Check sheet for the modelled part. Datum: model origin and axes. Units: mm. A direction names the side the tool comes from. Give positions to 0.01 mm unless a question says otherwise; leave off trailing zeros. Write each loop counter-clockwise with the first axis right and the second up, starting at its lowest first coordinate (ties: lowest second). Pieces come first, ordered by that corner, then holes.
from build123d import *

# Parameters (mm, degrees)
SKETCH1_W               = 28
SKETCH1_H               = 17.5
PCB_DEPTH               = 1.6
MOUNT_HOLE_1_DEPTH      = 34.057676869
MOUNT_HOLE_1_DEPTH_BACK = 34.057676869
SKETCH2_R               = 1.5
MOUNT_HOLE_2_DEPTH      = 34.057676869
MOUNT_HOLE_2_DEPTH_BACK = 34.057676869
SKETCH3_R               = 1.5
HEADER_10PIN_START      = 1.6
SKETCH4_W               = 25.4
SKETCH4_H               = 2.5
HEADER_10PIN_DEPTH      = 8.5
ADS1115_IC_START        = 1.6
SKETCH5_W               = 5
SKETCH5_H               = 3
ADS1115_IC_DEPTH        = 1
CAPS_START              = 1.6
SKETCH6_W               = 2
SKETCH6_H               = 1.2
CAPS_DEPTH              = 0.8


with BuildPart() as part:
    # Sketch1 → PCB (new body)
    with BuildSketch(Plane(origin=(0, 0, 0), x_dir=(1, 0, 0), z_dir=(0, 1, 0))):
        with Locations((14, 8.75)):
            Rectangle(SKETCH1_W, SKETCH1_H)
    extrude(amount=PCB_DEPTH)

    # Sketch2 → Mount_hole_1 (cut, two sides: drawn at the far end of the back side and taken through both)
    with BuildSketch(Plane(origin=(0, 0, 0), x_dir=(1, 0, 0), z_dir=(0, 1, 0)).offset(-MOUNT_HOLE_1_DEPTH_BACK)):
        with Locations(Location((2.5, 15, 0), (0, 0, 270))):
            Circle(SKETCH2_R)
    extrude(amount=MOUNT_HOLE_1_DEPTH + MOUNT_HOLE_1_DEPTH_BACK, mode=Mode.SUBTRACT)

    # Sketch3 → Mount_hole_2 (cut, two sides: drawn at the far end of the back side and taken through both)
    with BuildSketch(Plane(origin=(0, 0, 0), x_dir=(1, 0, 0), z_dir=(0, 1, 0)).offset(-MOUNT_HOLE_2_DEPTH_BACK)):
        with Locations(Location((25.5, 15, 0), (0, 0, 270))):
            Circle(SKETCH3_R)
    extrude(amount=MOUNT_HOLE_2_DEPTH + MOUNT_HOLE_2_DEPTH_BACK, mode=Mode.SUBTRACT)

    # Sketch4 → Header_10pin (add)
    with BuildSketch(Plane(origin=(0, 0, 0), x_dir=(1, 0, 0), z_dir=(0, 1, 0)).offset(HEADER_10PIN_START)):
        with Locations((14, 1.65)):
            Rectangle(SKETCH4_W, SKETCH4_H)
    extrude(amount=HEADER_10PIN_DEPTH)

    # Sketch5 → ADS1115_IC (add)
    with BuildSketch(Plane(origin=(0, 0, 0), x_dir=(1, 0, 0), z_dir=(0, 1, 0)).offset(ADS1115_IC_START)):
        with Locations((13.5, 8)):
            Rectangle(SKETCH5_W, SKETCH5_H)
    extrude(amount=ADS1115_IC_DEPTH)

    # Sketch6 → Caps (add)
    with BuildSketch(Plane(origin=(0, 0, 0), x_dir=(1, 0, 0), z_dir=(0, 1, 0)).offset(CAPS_START)):
        with Locations((18.5, 7.1)):
            Rectangle(SKETCH6_W, SKETCH6_H)
    extrude(amount=CAPS_DEPTH)


solid = part.part
1) Draft check along X on faces 1 (the flat face through (18, 2, -7.7)), 2 (the flat face through (17.5, 2, -7)), 3 (the flat face through (11, 2, -8)). Enter one of: +X half, -X half, draft (parallel to the pull), parting line (faces both ways), or undercut.
2) Sectioned sample at C-C on y = 1.25. Record the boundary of the cut face in (x, z), then the cut area to 3 significant figures.
3) Scan lines: L1, parallel to X at y = 0.5, z = -15; L2, parallel to Z at x = 2.5, y = 0.95; L3, parallel to Y at x = 11.75, z = -7.5. Record each from-to range of solid material in increasing order.
4) Gauge pin test, flat ends, axial feed: pin 1 (1.2 mm diameter, centred on y = 6, z = -1.5, fed in from -X); pin 2 (2.5 mm diameter, centred on x = 13.5, z = -7.5, fed in from +Y); pin 3 (0.6 mm diameter, centred on x = 18.5, z = -7, fed in from +Y); pin 4 (2.5 mm diameter, centred on x = 2.5, z = -15, fed in from +Y). Record the tip position at first contact, or that the pin passes through.
5) Access from +Z, -Z, +X, -X, +Y, -Y to the whole of each face (thin tool, end or side, straight path). Record for faces 4 (the flat face through (13, 2.6, -8)), 5 (the flat face through (19.5, 2, -7)), 6 (the flat face through (1.3, 6, -2)), 7 (the flat face through (14, 6, -0.4)), 8 (the flat face through (26.7, 6, -2)).
6) Sectioned sample at A-A on x = 2.5. Record the boundary of the cut face in (y, z).
7) Sectioned sample at D-D on x = 19. Record the boundary of the cut face in (y, z), then the cut area to 3 significant figures.
8) Sectioned sample at B-B on z = -15. Record the boundary of the cut face in (x, y), then the cut area to 3 significant figures.
Answers below:
1. face 1: draft
1. face 2: undercut
1. face 3: -X half
2. outline: (0, -17.5) - (28, -17.5) - (28, 0) - (0, 0) - close; hole circle Ø3 at (2.5, -15); hole circle Ø3 at (25.5, -15)
2. area: 476 mm2
3. L1: x = 0 to 1, 4 to 24, 27 to 28
3. L2: z = -17.5 to -16.5, -13.5 to 0
3. L3: y = 0 to 2.6
4. pin 1: stops at x = 1.3
4. pin 2: stops at y = 2.6
4. pin 3: stops at y = 2.4
4. pin 4: passes through
5. face 4: -Z, +X, -X, +Y
5. face 5: -Z, +X, +Y
5. face 6: +Z, -Z, -X, +Y
5. face 7: +Z, +X, -X, +Y
5. face 8: +Z, -Z, +X, +Y
6. outline: (0, -17.5) - (1.6, -17.5) - (1.6, -16.5) - (0, -16.5) - close; (0, -13.5) - (1.6, -13.5) - (1.6, -2.9) - (10.1, -2.9) - (10.1, -0.4) - (1.6, -0.4) - (1.6, 0) - (0, 0) - close
7. outline: (0, -17.5) - (1.6, -17.5) - (1.6, -7.7) - (2.4, -7.7) - (2.4, -6.5) - (1.6, -6.5) - (1.6, -2.9) - (10.1, -2.9) - (10.1, -0.4) - (1.6, -0.4) - (1.6, 0) - (0, 0) - close
7. area: 50.2 mm2
8. outline: (0, 0) - (1, 0) - (1, 1.6) - (0, 1.6) - close; (4, 0) - (24, 0) - (24, 1.6) - (4, 1.6) - close; (27, 0) - (28, 0) - (28, 1.6) - (27, 1.6) - close
8. area: 35.2 mm2
